Geometry check sheet. Reference: the model listing, model coordinates, mm. A direction names the side the tool comes from. Coordinates: 2 decimals unless noted, no trailing zeros. Write each loop counter-clockwise with the first axis right and the second up, starting at its lowest first coordinate (ties: lowest second). Pieces come first, ordered by that corner, then holes. Notation, with made-up numbers: (15, 31.25) -> (54, 31.25) arc R25 ccw to (54, 70.25) -> close; hole circle Ø9 at (35.25, 38.5). An arc over 180 degrees is marked (long way). Answer as CSV lines item,"result".
```python
from build123d import *

# Parameters (mm, degrees)
SKETCH1_W           = 19.05
SKETCH1_H           = 50.8
SKETCH1_R           = 3.175
BOSS_EXTRUDE1_DEPTH = 2.54
SKETCH2_W           = 19.05
SKETCH2_H           = 2.54
BOSS_EXTRUDE2_DEPTH = 50.8
BOSS_EXTRUDE5_DEPTH = 19.05
FILLET6_R           = 12.7
FILLET7_R           = 15.24
FILLET11_R          = 12.7
FILLET12_R          = 15.24


# Some blends are built 0.0001 mm under size
with BuildPart() as part:
    # Sketch1 → Boss-Extrude1 (new body)
    with BuildSketch(Plane.XY):
        with Locations((-165.075387597, 33.866666667)):
            Rectangle(SKETCH1_W, SKETCH1_H)
        with Locations((-165.075387597, 16.086666667)):
            Circle(SKETCH1_R, mode=Mode.SUBTRACT)
        with Locations((-165.075387597, 33.866666667)):
            Circle(SKETCH1_R, mode=Mode.SUBTRACT)
    extrude(amount=BOSS_EXTRUDE1_DEPTH)

    # Sketch2 → Boss-Extrude2 (add)
    with BuildSketch(Plane(origin=(0, 0, 0), x_dir=(-1, 0, 0), z_dir=(0, 0, -1))):
        with Locations((165.075387597, 57.996666667)):
            Rectangle(SKETCH2_W, SKETCH2_H)
    extrude(amount=BOSS_EXTRUDE2_DEPTH)

    # Sketch4 → Boss-Extrude5 (add)
    with BuildSketch(Plane(origin=(-155.550387597, 0, 0), x_dir=(0, 0, -1), z_dir=(1, 0, 0))):
        Polygon((48.26, 56.726666667), (48.26, 44.026666667), (78.74, 44.026666667), (78.74, 59.266666667), (76.2, 59.266666667), (76.2, 46.566666667), (50.8, 46.566666667), (50.8, 56.726666667), align=None)
    extrude(amount=-BOSS_EXTRUDE5_DEPTH)

    # Fillet6
    fillet6_edges = [part.edges().sort_by_distance(p)[0] for p in [
        (-165.075387597, 46.566666667, -50.8),
    ]]
    fillet(fillet6_edges, radius=FILLET6_R - 0.0001)  # a hair under: the kernel refuses the full size

    # Fillet7
    # the kernel refuses this fillet: 15.24 mm, written as the material it takes off along each edge
    with BuildSketch(Plane(origin=(-117.983280974, 44.026666667, -48.26), x_dir=(0, 0, -1), z_dir=(-1, 0, 0))) as fillet7_piece_1:
        with BuildLine():
            CenterArc((15.026842649, -15.24), FILLET7_R, 90, 80.405931773)
            Line((0, -12.7), (-0.300536853, -12.6492))
            ThreePointArc((-0.300536853, -12.6492), (-0.3048, -6.35), (-0.3048, 0))
            Line((-0.3048, 0), (0, 0.3048))
            Line((0, 0.3048), (15.026842649, 0.3048))
            Line((15.026842649, 0.3048), (15.026842649, 0))
        make_face()
    extrude(amount=94.184213245, mode=Mode.SUBTRACT)

    # Fillet11
    fillet11_edges = [part.edges().sort_by_distance(p)[0] for p in [
        (-165.075387597, 46.566666667, -76.2),
    ]]
    fillet(fillet11_edges, radius=FILLET11_R - 0.0001)  # a hair under: the kernel refuses the full size

    # Fillet12
    fillet12_edges = [part.edges().sort_by_distance(p)[0] for p in [
        (-165.075387597, 44.026666667, -78.74),
    ]]
    fillet(fillet12_edges, radius=FILLET12_R - 0.0001)  # a hair under: the kernel refuses the full size


solid = part.part
```
Item 1: Depth check by flat-ended pin: pin 1 Ø10 at (y, z) = (49, -24.5) entering from -X; pin 2 Ø3 at (x, z) = (-161, -14) entering from -Y; pin 3 Ø5 at (x, y) = (-168, 20.5) entering from -Z; pin 4 Ø10 at (x, z) = (-168.5, -65) entering from -Y. Enter the tip coordinate at first touch or a pass-through.
Responses:
pin 1,"passes through"
pin 2,"stops at y = 56.73"
pin 3,"stops at z = 0"
pin 4,"stops at y = 44.03"
Item 2: Set-up check for faces 1 (the flat face through (-165, 8.467, 1)), 2 (the cylindrical face through (-165.21, 50.39, -54.42)), 3 (the flat face through (-169, 33, 0)): record each of +Z, -Z, +X, -X, +Y, -Y from which the full face is reachable in a straight line by a thin tool's end or side.
Responses:
face 1,"+Z, -Z, +X, -X, -Y"
face 2,"+X, -X, +Y"
face 3,"+X, -X, -Y"
Item 3: Release check for a two-part mould opening along X. For faces 4 (the cylindrical face through (-162.047, 34.82, 1.252)), 5 (the cylindrical face through (-162.142, 14.871, 1.252)), 6 (the flat face through (-155.55, 58, -26)), 7 (the cylindrical face through (-165.21, 50.19, -72.38)) record: +X half, -X half, draft (parallel to the pull), parting line (faces both ways), or undercut.
Responses:
face 4,"undercut"
face 5,"undercut"
face 6,"+X half"
face 7,"draft"
Item 4: Cross-section at B-B, the plane x = -163.5. Count the separate pieces of the cut face and the enclosed holes in it, plus the area to 3 significant figures.
Responses:
separate pieces,"3"
enclosed holes,"0"
area,"338 mm2"
Item 5: Cross-section at A-A, the plane y = 35. Record the cut outline in (x, z), plus the area to 3 significant figures.
Responses:
outline,"(-174.6, 0) -> (-168.04, 0) -> (-168.04, 2.54) -> (-174.6, 2.54) -> close; (-162.11, 0) -> (-155.55, 0) -> (-155.55, 2.54) -> (-162.11, 2.54) -> close"
area,"33.3 mm2"
Item 6: Thickness scan on probe 1 along Z at (x, y) = (-168.25, 33); probe 2 along Y at (x, z) = (-165.75, -8.5); probe 3 along Z at (x, y) = (-161, 52). Record the ranges inside material, lowest first.
Responses:
probe 1,"z = 0 to 2.54"
probe 2,"y = 56.73 to 59.27"
probe 3,"z = -76.9 to -73.92, -53.08 to -49.89, 0 to 2.54"
